Build history of the part. All positions in model axes, mm. A direction names the side the tool comes from. Give positions to 0.01 mm unless a question says otherwise; leave off trailing zeros. Loops run counter-clockwise (first coordinate to the right, second up) from the corner with the lowest first, then second, coordinate; pieces in that order, holes last.
1) 3-axis set-ups, long thin cutter, end or side, ignore diameter. For faces 1 (the flat face through (4, -19, 20)), 2 (the flat face through (4, -55, 23)): which of +Z, -Z, +X, -X, +Y, -Y reach the whole face in a straight line?
2) Band-saw the part on A-A on y = -23. State how many separate pieces and enclosed holes the cut face has, then the cut area to 3 significant figures.
3) Wall check: line 1 (X direction, y = -23, z = 16) (3 decimals); line 2 (Y direction, x = -265, z = 14.5) (3 decimals); line 3 (Z direction, x = -72.5, y = -22). Give the ranges that are in metal, low to high.
4) Flat gauge pins, fed straight in: P1, Ø13, axis at x = 69, y = -24, coming from the +Z side; P2, Ø9, axis at x = 59.5, z = 23, coming from the -Y side. Where does each tip first touch, or does it go through?
5) Band-saw the part on B-B on x = 132.5. List the corners of the cut face in (y, z) (3 decimals).
6) Band-saw the part on C-C on x = -109.5. List the corners of the cut face in (y, z), then the cut area to 3 significant figures.
```python
from build123d import *

# Parameters (mm, degrees)
BOSS_EXTRUDE1_DEPTH                     = 290
TAP_DRILL_FOR_M10_HELICOIL1_D           = 10.25
TAP_DRILL_FOR_M10_HELICOIL1_CSINK_D     = 10.3
TAP_DRILL_FOR_M10_HELICOIL1_CSINK_ANGLE = 90


with BuildPart() as part:
    # Sketch1 → Boss-Extrude1 (new, symmetric)
    with BuildSketch(Plane(origin=(0, 0, 0), x_dir=(0, 0, -1), z_dir=(1, 0, 0))):
        with BuildLine():
            Line((0, 0), (-28, 0))
            Line((-28, 0), (-28, -15))
            Line((-28, -15), (-20, -15))
            Line((-20, -15), (-20, -31))
            Line((-20, -31), (-28, -31))
            Line((-28, -31), (-28, -50))
            Line((-28, -50), (-18, -60))
            Line((-18, -60), (-5, -60))
            ThreePointArc((-5, -60), (-1.464466094, -58.535533906), (0, -55))
            Line((0, -55), (0, 0))
        make_face()
    extrude(amount=BOSS_EXTRUDE1_DEPTH, both=True)

    # Tap Drill for M10 Helicoil1 (through all)
    with Locations(Plane(origin=(-265, -23, 20), x_dir=(1, 0, 0), z_dir=(0, 0, 1))):
        with Locations((0, 0), (132.5, 0), (265, 0), (397.5, 0), (530, 0)):
            CounterSinkHole(TAP_DRILL_FOR_M10_HELICOIL1_D / 2, TAP_DRILL_FOR_M10_HELICOIL1_CSINK_D / 2, counter_sink_angle=TAP_DRILL_FOR_M10_HELICOIL1_CSINK_ANGLE)


solid = part.part
```
Findings below:
1. face 1: +Z, +X, -X
1. face 2: +Z, +X, -X, -Y
2. separate pieces: 6
2. enclosed holes: 0
2. area: 10,600 mm2
3. line 1: x = -290 to -270.125, -259.875 to -137.625, -127.375 to -5.125, 5.125 to 127.375, 137.625 to 259.875, 270.125 to 290
3. line 2: y = -60 to -28.125, -17.875 to 0
3. line 3: z = 0 to 20
4. P1: stops at z = 20
4. P2: stops at y = -59.5
5. outline: (-60, 5) arc R5 ccw to (-55, 0) - (-28.125, 0) - (-28.125, 19.975) - (-28.15, 20) - (-31, 20) - (-31, 28) - (-50, 28) - (-60, 18) - close; (-17.875, 0) - (0, 0) - (0, 28) - (-15, 28) - (-15, 20) - (-17.85, 20) - (-17.875, 19.975) - close
6. outline: (-60, 5) arc R5 ccw to (-55, 0) - (0, 0) - (0, 28) - (-15, 28) - (-15, 20) - (-31, 20) - (-31, 28) - (-50, 28) - (-60, 18) - close
6. area: 1,500 mm2
